Autodesk Inventor part; units mm, degrees
ref_plane "YZ Plane" through (0, 0, 0) normal (1, 0, 0) x (0, 1, 0)
ref_plane "XZ Plane" through (0, 0, 0) normal (0, 1, 0) x (-1, 0, 0)
ref_plane "XY Plane" through (0, 0, 0) normal (0, 0, 1) x (1, 0, 0)
sketch "Sketch1" plane through (0, 0, 0) normal (0, 1, 0) x (-1, 0, 0)
  arc A0 (-42.1977, 20.587) -> (-43.9298, 19.587) centre (-42.1977, 18.587) ccw
  line L0 (-45.9298, 17.587) -> (-43.9298, 19.587)
  line L1 (-50.9298, 12.587) -> (-45.9298, 17.587)
  line L2 (-50.9298, -22.413) -> (-50.9298, 12.587)
  line L3 (-43.9298, -29.413) -> (-50.9298, -22.413)
  arc A1 (-43.9298, -29.413) -> (-42.1977, -30.413) centre (-42.1977, -28.413) ccw
  line L4 (-32.6618, -30.413) -> (-42.1977, -30.413)
  arc A2 (-32.6618, -30.413) -> (-30.9298, -29.413) centre (-32.6618, -28.413) ccw
  line L5 (-28.9298, -27.413) -> (-30.9298, -29.413)
  line L6 (-20.9298, -27.413) -> (-28.9298, -27.413)
  line L7 (-18.9298, -29.413) -> (-20.9298, -27.413)
  arc A3 (-18.9298, -29.413) -> (-17.1977, -30.413) centre (-17.1977, -28.413) ccw
  line L8 (-7.6618, -30.413) -> (-17.1977, -30.413)
  arc A4 (-7.6618, -30.413) -> (-5.9298, -29.413) centre (-7.6618, -28.413) ccw
  line L9 (-3.9298, -27.413) -> (-5.9298, -29.413)
  line L10 (4.0702, -27.413) -> (-3.9298, -27.413)
  line L11 (6.0702, -29.413) -> (4.0702, -27.413)
  arc A5 (6.0702, -29.413) -> (7.8023, -30.413) centre (7.8023, -28.413) ccw
  line L12 (17.3382, -30.413) -> (7.8023, -30.413)
  arc A6 (17.3382, -30.413) -> (19.0702, -29.413) centre (17.3382, -28.413) ccw
  line L13 (21.0702, -27.413) -> (19.0702, -29.413)
  line L14 (29.0702, -27.413) -> (21.0702, -27.413)
  line L15 (31.0702, -29.413) -> (29.0702, -27.413)
  arc A7 (31.0702, -29.413) -> (32.8023, -30.413) centre (32.8023, -28.413) ccw
  line L16 (42.3382, -30.413) -> (32.8023, -30.413)
  arc A8 (42.3382, -30.413) -> (44.0702, -29.413) centre (42.3382, -28.413) ccw
  line L17 (46.0702, -27.413) -> (44.0702, -29.413)
  line L18 (49.0702, -27.413) -> (46.0702, -27.413)
  line L19 (59.0702, -17.413) -> (49.0702, -27.413)
  line L20 (59.0702, 7.587) -> (59.0702, -17.413)
  line L21 (49.0702, 17.587) -> (59.0702, 7.587)
  line L22 (46.0702, 17.587) -> (49.0702, 17.587)
  line L23 (44.0702, 19.587) -> (46.0702, 17.587)
  arc A9 (44.0702, 19.587) -> (42.3382, 20.587) centre (42.3382, 18.587) ccw
  line L24 (32.8023, 20.587) -> (42.3382, 20.587)
  arc A10 (32.8023, 20.587) -> (31.0702, 19.587) centre (32.8023, 18.587) ccw
  line L25 (29.0702, 17.587) -> (31.0702, 19.587)
  line L26 (21.0702, 17.587) -> (29.0702, 17.587)
  line L27 (19.0702, 19.587) -> (21.0702, 17.587)
  arc A11 (19.0702, 19.587) -> (17.3382, 20.587) centre (17.3382, 18.587) ccw
  line L28 (7.8023, 20.587) -> (17.3382, 20.587)
  arc A12 (7.8023, 20.587) -> (6.0702, 19.587) centre (7.8023, 18.587) ccw
  line L29 (4.0702, 17.587) -> (6.0702, 19.587)
  line L30 (-3.9298, 17.587) -> (4.0702, 17.587)
  line L31 (-5.9298, 19.587) -> (-3.9298, 17.587)
  arc A13 (-5.9298, 19.587) -> (-7.6618, 20.587) centre (-7.6618, 18.587) ccw
  line L32 (-17.1977, 20.587) -> (-7.6618, 20.587)
  arc A14 (-17.1977, 20.587) -> (-18.9298, 19.587) centre (-17.1977, 18.587) ccw
  line L33 (-20.9298, 17.587) -> (-18.9298, 19.587)
  line L34 (-28.9298, 17.587) -> (-20.9298, 17.587)
  line L35 (-30.9298, 19.587) -> (-28.9298, 17.587)
  arc A15 (-30.9298, 19.587) -> (-32.6618, 20.587) centre (-32.6618, 18.587) ccw
  line L36 (-42.1977, 20.587) -> (-32.6618, 20.587)
  point P0 (0, 0)
  point P1 (59.0702, 17.587)
extrude "Extrusion1" add sketch "Sketch1" along normal blind 2
sketch "Sketch2" plane through (0, 2, 0) normal (0, 1, 0) x (1, 0, 0)
  line L0 (-21.0702, 27.413) -> (-29.0702, 27.413)
  line L1 (-28.7702, 22.413) -> (-28.7702, 15.413)
  line L2 (-21.0023, 22.413) -> (-21.0023, 15.413)
  line L3 (-28.7702, -5.587) -> (-28.7702, -12.587)
  line L4 (-21.0023, -5.587) -> (-21.0023, -12.587)
  line L5 (-37.2702, -5.587) -> (-28.7702, -5.587)
  line L6 (-21.0023, -5.587) -> (-12.5023, -5.587)
  line L7 (-12.5023, 15.413) -> (-21.0023, 15.413)
  line L8 (-28.7702, 15.413) -> (-37.2702, 15.413)
  line L9 (-37.2702, 22.413) -> (-28.7702, 22.413)
  line L10 (-21.0023, 22.413) -> (-12.5023, 22.413)
  line L11 (-12.5023, -12.587) -> (-21.0023, -12.587)
  line L12 (-28.7702, -12.587) -> (-37.2702, -12.587)
  line L13 (-37.2702, -12.587) -> (-37.2702, -5.587)
  line L14 (-37.2702, 15.413) -> (-37.2702, 22.413)
  line L15 (-12.5023, 22.413) -> (-12.5023, 15.413)
  line L16 (-12.5023, -5.587) -> (-12.5023, -12.587)
  line L17 (-29.0702, -17.587) -> (-21.0702, -17.587)
  line L18 (-49.0702, -17.587) -> (-46.0702, -17.587)
  arc A0 (42.1977, -20.587) -> (43.9298, -19.587) centre (42.1977, -18.587) ccw
  point P0 (0, 0)
  point P1 (-47.5702, -17.587)
  point P2 (43.1977, -20.319)
  dimension "d15" = 8.5
  dimension "d16" = 8.5
  dimension "d19" = 10.3
  dimension "d22" = 55.7
  dimension "d23" = 5
  dimension "d24" = 5
  dimension "d25" = 5
  dimension "d26" = 5
  dimension "d27" = 7
extrude "Extrusion4" cut sketch "Sketch2" against normal blind 10
sketch "Sketch4" plane through (0, 0, 0) normal (0, -1, 0) x (1, 0, 0)
  line L0 (-49.0702, 17.587) -> (-46.0702, 17.587)
  line L1 (28.9298, 17.587) -> (30.9298, 19.587)
  line L2 (-46.0702, 17.587) -> (45.9298, 17.587)
  line L3 (43.9298, 19.587) -> (50.9298, 12.587)
  line L4 (-44.0702, -29.413) -> (-46.0702, -27.413)
  line L5 (-46.0702, -27.413) -> (45.9298, -27.413)
  line L6 (50.9298, -22.413) -> (43.9298, -29.413)
  line L7 (-46.0702, 17.587) -> (-49.0702, 17.587)
  line L8 (-59.0702, 7.587) -> (-49.0702, 17.587)
  line L9 (-49.0702, 17.587) -> (-59.0702, 7.587)
  line L10 (-59.0702, -17.413) -> (-59.0702, 7.587)
  line L11 (-59.0702, 7.587) -> (-59.0702, -17.413)
  line L12 (-59.0702, -17.413) -> (-49.0702, -27.413)
  line L13 (-49.0702, -27.413) -> (-46.0702, -27.413)
  line L14 (45.9298, 17.587) -> (50.9298, 12.587)
  line L15 (50.9298, 12.587) -> (50.9298, -22.413)
  line L16 (50.9298, -22.413) -> (45.9298, -27.413)
  line L17 (50.9298, 12.587) -> (50.9298, -22.413)
  line L18 (-37.2702, -15.413) -> (-28.7702, -15.413)
  line L19 (-28.7702, -15.413) -> (-28.7702, -22.413)
  line L20 (-28.7702, -22.413) -> (-37.2702, -22.413)
  line L21 (-37.2702, -22.413) -> (-37.2702, -15.413)
  line L22 (-37.2702, 12.587) -> (-28.7702, 12.587)
  line L23 (-28.7702, 12.587) -> (-28.7702, 5.587)
  line L24 (-28.7702, 5.587) -> (-37.2702, 5.587)
  line L25 (-37.2702, 5.587) -> (-37.2702, 12.587)
  line L26 (-21.0023, -15.413) -> (-12.5023, -15.413)
  line L27 (-12.5023, -15.413) -> (-12.5023, -22.413)
  line L28 (-12.5023, -22.413) -> (-21.0023, -22.413)
  line L29 (-21.0023, -22.413) -> (-21.0023, -15.413)
  line L30 (-21.0023, 12.587) -> (-12.5023, 12.587)
  line L31 (-12.5023, 12.587) -> (-12.5023, 5.587)
  line L32 (-12.5023, 5.587) -> (-21.0023, 5.587)
  line L33 (-21.0023, 5.587) -> (-21.0023, 12.587)
  line L34 (17.1977, -30.413) -> (7.6618, -30.413)
  arc A0 (17.1977, -30.413) -> (18.9298, -29.413) centre (17.1977, -28.413) ccw
  line L35 (20.9298, -27.413) -> (18.9298, -29.413)
  line L36 (28.9298, -27.413) -> (20.9298, -27.413)
  line L37 (30.9298, -29.413) -> (28.9298, -27.413)
  arc A1 (30.9298, -29.413) -> (32.6618, -30.413) centre (32.6618, -28.413) ccw
  line L38 (42.1977, -30.413) -> (32.6618, -30.413)
  arc A2 (42.1977, -30.413) -> (43.9298, -29.413) centre (42.1977, -28.413) ccw
  line L39 (50.9298, -22.413) -> (43.9298, -29.413)
  line L40 (50.9298, 12.587) -> (50.9298, -22.413)
  line L41 (43.9298, 19.587) -> (50.9298, 12.587)
  arc A3 (43.9298, 19.587) -> (42.1977, 20.587) centre (42.1977, 18.587) ccw
  line L42 (32.6618, 20.587) -> (42.1977, 20.587)
  arc A4 (32.6618, 20.587) -> (30.9298, 19.587) centre (32.6618, 18.587) ccw
  line L43 (28.9298, 17.587) -> (30.9298, 19.587)
  line L44 (20.9298, 17.587) -> (28.9298, 17.587)
  line L45 (18.9298, 19.587) -> (20.9298, 17.587)
  arc A5 (18.9298, 19.587) -> (17.1977, 20.587) centre (17.1977, 18.587) ccw
  line L46 (7.6618, 20.587) -> (17.1977, 20.587)
  arc A6 (7.6618, 20.587) -> (5.9298, 19.587) centre (7.6618, 18.587) ccw
  line L47 (3.9298, 17.587) -> (5.9298, 19.587)
  line L48 (-4.0702, 17.587) -> (3.9298, 17.587)
  line L49 (-6.0702, 19.587) -> (-4.0702, 17.587)
  arc A7 (-6.0702, 19.587) -> (-7.8023, 20.587) centre (-7.8023, 18.587) ccw
  line L50 (-17.3382, 20.587) -> (-7.8023, 20.587)
  arc A8 (-17.3382, 20.587) -> (-19.0702, 19.587) centre (-17.3382, 18.587) ccw
  line L51 (-21.0702, 17.587) -> (-19.0702, 19.587)
  line L52 (-29.0702, 17.587) -> (-21.0702, 17.587)
  line L53 (-31.0702, 19.587) -> (-29.0702, 17.587)
  arc A9 (-31.0702, 19.587) -> (-32.8023, 20.587) centre (-32.8023, 18.587) ccw
  line L54 (-42.3382, 20.587) -> (-32.8023, 20.587)
  arc A10 (-42.3382, 20.587) -> (-44.0702, 19.587) centre (-42.3382, 18.587) ccw
  line L55 (-46.0702, 17.587) -> (-44.0702, 19.587)
  line L56 (-49.0702, 17.587) -> (-46.0702, 17.587)
  line L57 (-59.0702, 7.587) -> (-49.0702, 17.587)
  line L58 (-59.0702, -17.413) -> (-59.0702, 7.587)
  line L59 (-49.0702, -27.413) -> (-59.0702, -17.413)
  line L60 (-46.0702, -27.413) -> (-49.0702, -27.413)
  line L61 (-44.0702, -29.413) -> (-46.0702, -27.413)
  arc A11 (-44.0702, -29.413) -> (-42.3382, -30.413) centre (-42.3382, -28.413) ccw
  line L62 (-32.8023, -30.413) -> (-42.3382, -30.413)
  arc A12 (-32.8023, -30.413) -> (-31.0702, -29.413) centre (-32.8023, -28.413) ccw
  line L63 (-29.0702, -27.413) -> (-31.0702, -29.413)
  line L64 (-21.0702, -27.413) -> (-29.0702, -27.413)
  line L65 (-19.0702, -29.413) -> (-21.0702, -27.413)
  arc A13 (-19.0702, -29.413) -> (-17.3382, -30.413) centre (-17.3382, -28.413) ccw
  line L66 (-7.8023, -30.413) -> (-17.3382, -30.413)
  arc A14 (-7.8023, -30.413) -> (-6.0702, -29.413) centre (-7.8023, -28.413) ccw
  line L67 (-4.0702, -27.413) -> (-6.0702, -29.413)
  line L68 (3.9298, -27.413) -> (-4.0702, -27.413)
  line L69 (5.9298, -29.413) -> (3.9298, -27.413)
  arc A15 (5.9298, -29.413) -> (7.6618, -30.413) centre (7.6618, -28.413) ccw
  point P0 (0, 0)
extrude "Extrusion6" add sketch "Sketch4" along normal blind 0.01 contours L0 L2 L3 L15 L6 L5 L13 L12 L10 L8
sketch "Sketch5" plane through (0, -0.01, 0) normal (0, -1, 0) x (1, 0, 0)
  line L0 (50.9298, 12.587) -> (45.9298, 17.587)
  line L1 (45.9298, 17.587) -> (-49.0702, 17.587)
  line L2 (-49.0702, 17.587) -> (-59.0702, 7.587)
  line L3 (-59.0702, 7.587) -> (-59.0702, -17.413)
  line L4 (-59.0702, -17.413) -> (-49.0702, -27.413)
  line L5 (-49.0702, -27.413) -> (45.9298, -27.413)
  line L6 (45.9298, -27.413) -> (50.9298, -22.413)
  line L7 (50.9298, -22.413) -> (50.9298, 12.587)
  line L8 (-37.2702, -15.413) -> (-28.7702, -15.413)
  line L9 (-28.7702, -15.413) -> (-28.7702, -22.413)
  line L10 (-28.7702, -22.413) -> (-37.2702, -22.413)
  line L11 (-37.2702, -22.413) -> (-37.2702, -15.413)
  line L12 (-37.2702, 12.587) -> (-28.7702, 12.587)
  line L13 (-28.7702, 12.587) -> (-28.7702, 5.587)
  line L14 (-28.7702, 5.587) -> (-37.2702, 5.587)
  line L15 (-37.2702, 5.587) -> (-37.2702, 12.587)
  line L16 (-21.0023, -15.413) -> (-12.5023, -15.413)
  line L17 (-12.5023, -15.413) -> (-12.5023, -22.413)
  line L18 (-12.5023, -22.413) -> (-21.0023, -22.413)
  line L19 (-21.0023, -22.413) -> (-21.0023, -15.413)
  line L20 (-21.0023, 12.587) -> (-12.5023, 12.587)
  line L21 (-12.5023, 12.587) -> (-12.5023, 5.587)
  line L22 (-12.5023, 5.587) -> (-21.0023, 5.587)
  line L23 (-21.0023, 5.587) -> (-21.0023, 12.587)
  line L24 (44, -24.913) -> (-48.0347, -24.913)
  line L25 (-48.0347, -24.913) -> (-56.5702, -16.3775)
  line L26 (-56.5702, -16.3775) -> (-56.5702, 6.5514)
  line L27 (-56.5702, 6.5514) -> (-48.0347, 15.087)
  line L28 (-48.0347, 15.087) -> (44, 15.087)
  line L29 (48.4298, 10.8192) -> (48.4298, -20.6453)
  line L30 (-57.5702, -16.7917) -> (-57.5702, 6.9656)
  line L31 (-57.5702, 6.9656) -> (-48.4489, 16.087)
  line L32 (-48.4489, 16.087) -> (44, 16.087)
  line L33 (49.4298, 10.8192) -> (49.4298, -20.6453)
  line L34 (44, -25.913) -> (-48.4489, -25.913)
  line L35 (-48.4489, -25.913) -> (-57.5702, -16.7917)
  line L36 (44, 15.087) -> (44, 16.087)
  line L37 (44, -24.913) -> (44, -25.913)
  line L38 (49.4298, -20.6453) -> (48.4298, -20.6453)
  line L39 (49.4298, 10.8192) -> (48.4298, 10.8192)
  point P0 (0, 0)
  dimension "d34" = 2.5
  dimension "d35" = 1.5
extrude "Extrusion7" add sketch "Sketch5" along normal blind 2 contours L37 L34 L35 L30 L31 L32 L36 L28 L27 L26 L25 L24 | L39 L33 L38 L29
sketch "Sketch6" plane through (-57.5702, -0.01, -16.7917) normal (-1, 0, 0) x (0, 0, 1)
  line L0 (27.6109, -2) -> (-3.8536, -2)
  line L1 (5, 0) -> (18.7574, 0)
  line L2 (18.7574, 0) -> (18.7574, -2)
  line L3 (18.7574, -2) -> (5, -2)
  line L4 (5, -2) -> (5, 0)
  line L5 (0, 0) -> (0, -2)
  line L6 (23.7574, 0) -> (23.7574, -2)
  point P0 (16.7917, 0.01)
  point P1 (28.3431, -2)
  point P2 (-4.5858, -2)
  dimension "d38" = 5
  dimension "d39" = 5
extrude "Extrusion8" cut sketch "Sketch6" against normal blind 2
properties part number "RC5 Controller kryt"
Design review of the part built by this model. Coordinates are the model's own, in mm. A direction names the side the tool comes from. Round coordinates to 2 decimals unless told otherwise and drop trailing zeros. Loops run counter-clockwise (first coordinate to the right, second up) from the corner with the lowest first, then second, coordinate; pieces in that order, holes last. Notation, with made-up numbers: (-31.5, 38) -> (4.5, 38) arc R13 cw to (4.5, 43) -> close; hole circle Ø3 at (-29.5, 54). An arc over 180 degrees is marked (long way). Use one line per item in the form item = value. Start each with the question number.
Q1. For pin 1 Ø1 at (y, z) = (1, -19.5) entering from -X; pin 2 Ø0.6 at (x, y) = (-19.5, -1) entering from -Z; pin 3 Ø0.9 at (x, z) = (40.5, -29) entering from -Y, all flat-tipped, find the tip position at first contact; note any pin that passes through.
Q2. Wall thickness on line 1 along Z through (x, y) = (-29, 1.5); line 2 along X through (y, z) = (-0.45, 6.5); line 3 along X through (y, z) = (1.35, -20.5): over which ranges is each line inside the solid? List them lowest first. Write a range as [from, to].
Q3. Draft analysis for pull direction X (two halves, no side actions). For faces 5 (the face through (-33, 1, -15.413)), 6 (the face through (-54.14, 1.009, -22.343)), 7 (the face through (-3, 2, -5)), state which applies: +X half, -X half, draft (parallel to the pull), parting line (faces both ways), or undercut.
Q4. We need section A-A on y = -1.25. Give the boundary of the cut face in (x, z).
Q5. We need section D-D on z = -4.5. Give the boundary of the cut face in (x, y), then the cut area to 3 significant figures.
Q6. We need section B-B on z = -19.5. Give the boundary of the cut face in (x, y).
Q7. Machinability: for faces 1 (the face through (-52.946, -0.996, -21.416)), 2 (the face through (-56.57, -1, -14)), 3 (the face through (-1, -1, -24.913)), 4 (the face through (-28.77, 1, 9)), which of the approach directions +Z, -Z, +X, -X, +Y, -Y give a long, thin tool a straight path to every point of the face, cutting with its end or side? Answer none if there is none.
Calculated:
q1.pin_1 = -57.48
q1.pin_2 = -25.91
q1.pin_3 = 0
q2.line_1 = [-27.41, -22.41], [-15.41, 5.59], [12.59, 17.59]
q2.line_2 = [-57.57, -56.57], [48.43, 49.43]
q2.line_3 = [-55.98, -37.27], [-28.77, -21], [-12.5, 50.93]
q3.face_5 = undercut
q3.face_6 = -X half
q3.face_7 = draft
q4.outline = (-57.57, -16.79) -> (-48.45, -25.91) -> (44, -25.91) -> (44, -24.91) -> (-48.03, -24.91) -> (-56.57, -16.38) -> (-56.57, -11.79) -> (-57.57, -11.79) -> close; (-57.57, 1.97) -> (-56.57, 1.97) -> (-56.57, 6.55) -> (-48.03, 15.09) -> (44, 15.09) -> (44, 16.09) -> (-48.45, 16.09) -> (-57.57, 6.97) -> close; (48.43, -20.65) -> (49.43, -20.65) -> (49.43, 10.82) -> (48.43, 10.82) -> close
q5.outline = (-59.07, -0.01) -> (48.43, -0.01) -> (48.43, -2.01) -> (49.43, -2.01) -> (49.43, -0.01) -> (50.93, -0.01) -> (50.93, 2) -> (-59.07, 2) -> close
q5.area = 223 mm²
q6.outline = (-56.98, -0.01) -> (-54.86, -0.01) -> (-54.86, -2.01) -> (-53.45, -2.01) -> (-53.45, -0.01) -> (-37.27, -0.01) -> (-37.27, 2) -> (-56.98, 2) -> close; (-28.77, -0.01) -> (-21, -0.01) -> (-21, 2) -> (-28.77, 2) -> close; (-12.5, -0.01) -> (48.43, -0.01) -> (48.43, -2.01) -> (49.43, -2.01) -> (49.43, -0.01) -> (50.93, -0.01) -> (50.93, 2) -> (-12.5, 2) -> close
q7.face_1 = -Z, -X, -Y
q7.face_2 = -Y
q7.face_3 = +X, -Y
q7.face_4 = +Y, -Y
